Work out the finished part from the listing and answer in its coordinate system (mm). A direction names the side the tool comes from. Give positions to 0.01 mm unless a question says otherwise; leave off trailing zeros. Loops run counter-clockwise (first coordinate to the right, second up) from the corner with the lowest first, then second, coordinate; pieces in that order, holes last. Notation, with made-up numbers: (21.5, -4) - (46.5, -4) arc R26 ccw to (46.5, 25) - close; hole circle Ø6 at (-21, 13.5). An arc over 180 degrees is marked (long way). Use CSV: the item, a comma, the result in double quotes.
from build123d import *

# Parameters (mm, degrees)
SKETCH1_W           = 104
SKETCH1_H           = 104
SKETCH1_R           = 25
BOSS_EXTRUDE1_DEPTH = 115
CUT_EXTRUDE3_DEPTH  = 115
CUT_EXTRUDE4_DEPTH  = 115
CUT_EXTRUDE5_DEPTH  = 116
FILLET1_R           = 10
SKETCH9_R           = 35
CUT_EXTRUDE6_DEPTH  = 10
SKETCH10_R          = 35
CUT_EXTRUDE7_DEPTH  = 10
BOSS_EXTRUDE2_DEPTH = 10
FILLET2_R           = 5
CUT_EXTRUDE8_DEPTH  = 10


with BuildPart() as part:
    # Sketch1 → Boss-Extrude1 (new body)
    with BuildSketch(Plane.XY):
        Rectangle(SKETCH1_W, SKETCH1_H)
        Circle(SKETCH1_R, mode=Mode.SUBTRACT)
    extrude(amount=BOSS_EXTRUDE1_DEPTH)

    # Sketch7 → Cut-Extrude3 (cut)
    with BuildSketch(Plane.ZY.offset(52)):
        Polygon((0, 52), (115, 52), (57.5, 27.592698068), align=None)
        Polygon((0, -52), (115, -52), (57.5, -27.592698068), align=None)
    extrude(amount=-CUT_EXTRUDE3_DEPTH, mode=Mode.SUBTRACT)

    # Sketch4 → Cut-Extrude4 (cut)
    with BuildSketch(Plane(origin=(0, 52, 0), x_dir=(1, 0, 0), z_dir=(0, 1, 0))):
        Polygon((-52, 0), (-27.592698068, -57.5), (-52, -115), align=None)
        Polygon((52, -115), (27.592698068, -57.5), (52, 0), align=None)
    extrude(amount=-CUT_EXTRUDE4_DEPTH, mode=Mode.SUBTRACT)

    # Sketch8 → Cut-Extrude5 (cut, through all)
    with BuildSketch(Plane(origin=(0, 0, 0), x_dir=(-1, 0, 0), z_dir=(0, 0, -1))):
        with BuildLine():
            Line((0, 0), (96.389790508, 0))
            ThreePointArc((96.389790508, 0), (83.425867148, -83.299633305), (0, -95.424686222))
            Line((0, -95.424686222), (0, 0))
        make_face()
    extrude(amount=-CUT_EXTRUDE5_DEPTH, mode=Mode.SUBTRACT)

    # Fillet1
    fillet1_edges = [part.edges().sort_by_distance(p)[0] for p in [
        (13.796349034, -27.592698068, 57.5),
        (0, 27.592698068, 57.5),
        (27.592698068, 0, 57.5),
        (-27.592698068, 13.796349034, 57.5),
    ]]
    fillet(fillet1_edges, radius=FILLET1_R)

    # Sketch9 → Cut-Extrude6 (cut)
    with BuildSketch(Plane(origin=(0, 0, 0), x_dir=(-1, 0, 0), z_dir=(0, 0, -1))):
        Circle(SKETCH9_R)
    extrude(amount=-CUT_EXTRUDE6_DEPTH, mode=Mode.SUBTRACT)

    # Sketch10 → Cut-Extrude7 (cut)
    with BuildSketch(Plane.XY.offset(115)):
        Circle(SKETCH10_R)
    extrude(amount=-CUT_EXTRUDE7_DEPTH, mode=Mode.SUBTRACT)

    # Sketch11 → Boss-Extrude2 (add)
    with BuildSketch(Plane(origin=(0, 0, 0), x_dir=(-1, 0, 0), z_dir=(0, 0, -1))):
        Polygon((52, 0), (52, 52), (-52, 52), (-52, -52), (0, -52), (0, -49), (-49, -49), (-49, 49), (49, 49), (49, 0), align=None)
    extrude(amount=BOSS_EXTRUDE2_DEPTH)

    # Fillet2
    fillet2_edges = [part.edges().sort_by_distance(p)[0] for p in [
        (0, 52, 0),
        (52, 0, 0),
        (-52, 26, 0),
        (26, -52, 0),
    ]]
    fillet(fillet2_edges, radius=FILLET2_R)

    # Sketch12 → Cut-Extrude8 (cut)
    with BuildSketch(Plane(origin=(0, 0, 0), x_dir=(-1, 0, 0), z_dir=(0, 0, -1))):
        with BuildLine():
            Line((27.930717857, 32.173358544), (38.537319575, 42.779960262))
            ThreePointArc((38.537319575, 42.779960262), (42.779960262, 42.779960262), (42.779960262, 38.537319575))
            Line((42.779960262, 38.537319575), (32.173358544, 27.930717857))
            ThreePointArc((32.173358544, 27.930717857), (27.930717857, 27.930717857), (27.930717857, 32.173358544))
        make_face()
        with BuildLine():
            Line((-32.173358544, 27.930717857), (-42.779960262, 38.537319575))
            ThreePointArc((-42.779960262, 38.537319575), (-42.779960262, 42.779960262), (-38.537319575, 42.779960262))
            Line((-38.537319575, 42.779960262), (-27.930717857, 32.173358544))
            ThreePointArc((-27.930717857, 32.173358544), (-27.930717857, 27.930717857), (-32.173358544, 27.930717857))
        make_face()
        with BuildLine():
            Line((-27.930717857, -32.173358544), (-38.537319575, -42.779960262))
            ThreePointArc((-38.537319575, -42.779960262), (-42.779960262, -42.779960262), (-42.779960262, -38.537319575))
            Line((-42.779960262, -38.537319575), (-32.173358544, -27.930717857))
            ThreePointArc((-32.173358544, -27.930717857), (-27.930717857, -27.930717857), (-27.930717857, -32.173358544))
        make_face()
    extrude(amount=-CUT_EXTRUDE8_DEPTH, mode=Mode.SUBTRACT)


solid = part.part
Item 1: Given P1, Ø18.5, axis at x = -36, y = 38, coming from the -Z side; P2, Ø12, axis at y = -9.5, z = 77, coming from the -X side; P3, Ø8, axis at x = -12, z = -6, coming from the -Y side, each flat-ended and moving along its own axis, determine where each tip first touches the part or whether it passes through.
Determined:
P1,"stops at z = 0"
P2,"stops at x = 19.62"
P3,"stops at y = 49"
Item 2: The mould has two halves that part along Y. Classify faces 1 (the flat face through (19.71, -40.27, 27.63)), 2 (the cylindrical face through (27.98, -27.88, 4.93)), 3 (the flat face through (-40.58, 20.43, 26.9)), 4 (the cylindrical face through (-27.98, 27.88, 4.93)): pulls with the +Y half, pulls with the -Y half, needs draft (parallel to the pull), parting line crosses it, or undercut.
Determined:
face 1,"pulls with the -Y half"
face 2,"undercut"
face 3,"needs draft"
face 4,"undercut"
Item 3: A cutting plane is placed at A-A on x = 16. Determine the outline of the cut face in (y, z).
Determined:
outline,"(-52, -10) - (-49, -10) - (-49, 0) - (-31.13, 0) - (-31.13, 10) - (-19.21, 10) - (-19.21, 105) - (-31.13, 105) - (-31.13, 115) - (-52, 115) - (-29.25, 61.41) arc R10 cw to (-29.25, 53.59) - (-51.6, 0.94) arc R5 ccw to (-52, -1.02) - close; (19.21, 10) - (31.13, 10) - (31.13, 0) - (49, 0) - (49, -10) - (52, -10) - (52, -1.02) arc R5 ccw to (51.6, 0.94) - (29.25, 53.59) arc R10 cw to (29.25, 61.41) - (52, 115) - (31.13, 115) - (31.13, 105) - (19.21, 105) - close"
Item 4: A cutting plane is placed at C-C on y = -23. Determine the outline of the cut face in (x, z), and give its area (3 significant figures).
Determined:
outline,"(9.8, 10) - (26.38, 10) - (26.38, 0) - (49, 0) - (49, -10) - (52, -10) - (52, -1.02) arc R5 ccw to (51.6, 0.94) - (29.25, 53.59) arc R10 cw to (29.25, 61.41) - (52, 115) - (26.38, 115) - (26.38, 105) - (9.8, 105) - close"
area,"3,150 mm²"
Item 5: A cutting plane is placed at D-D on z = 46. Determine the outline of the cut face in (x, y).
Determined:
outline,"(-32.47, 0) - (-25, 0) arc R25 cw (long way) to (0, -25) - (0, -32.47) - (32.47, -32.47) - (32.47, 32.47) - (-32.47, 32.47) - close"
Item 6: Find the intervals of material crossed by line 1 (Z direction, x = 18, y = 20.5); line 2 (Z direction, x = 37, y = 21.5); line 3 (Z direction, x = 23.5, y = 39.5), in increasing order.
Determined:
line 1,"z = 10 to 105"
line 2,"z = 0 to 35.34, 79.66 to 115"
line 3,"z = 0 to 29.45, 85.55 to 115"
Item 7: For faces 5 (the flat face through (-37.55, 33.31, 4.93)), 6 (the flat face through (24, -49, -5)), 7 (the cylindrical face through (25.55, 23.92, 110.07)), 8 (the flat face through (19.858, -40.785, 88.579)), determine the directions among +Z, -Z, +X, -X, +Y, -Y from which every point of the face is accessible in a straight line to the end or side of a thin tool.
Determined:
face 5,"-Z"
face 6,"-Z, -X"
face 7,"+Z"
face 8,"+X, -X, -Y"
Item 8: A cutting plane is placed at B-B on z = 7.5. Determine the outline of the cut face in (x, y), and give its area (3 significant figures).
Determined:
outline,"(-48.82, 0) - (-35, 0) arc R35 cw (long way) to (0, -35) - (0, -48.82) - (48.82, -48.82) - (48.82, 48.82) - (-48.82, 48.82) - close; hole (-42.78, 38.54) - (-32.17, 27.93) arc R3 ccw to (-27.93, 32.17) - (-38.54, 42.78) arc R3 ccw to start; hole (27.93, -32.17) - (38.54, -42.78) arc R3 ccw to (42.78, -38.54) - (32.17, -27.93) arc R3 ccw to start; hole (27.93, 32.17) arc R3 ccw to (32.17, 27.93) - (42.78, 38.54) arc R3 ccw to (38.54, 42.78) - close"
area,"3,910 mm²"
